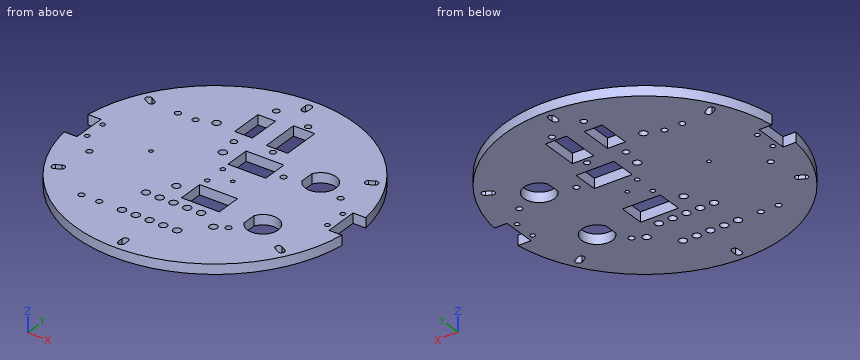
```python
from build123d import *

# Parameters (mm, degrees)
ESQUISSE1_R                     = 71
BOSS_EXTRU_1_DEPTH              = 5
ESQUISSE2_W                     = 33.992340046
ESQUISSE2_H                     = 17
ESQUISSE2_W_2                   = 21.861356716
ENL_V_MAT_EXTRU_1_DEPTH         = 101.533576481
D_GAGEMENT_M21_D                = 2.4
R_P_TITION_LIN_AIRE1_COUNT      = 3
R_P_TITION_LIN_AIRE1_PITCH      = 61
R_P_TITION_LIN_AIRE1_COUNT_DIR2 = 2
R_P_TITION_LIN_AIRE1_PITCH_DIR2 = 11
ESQUISSE7_R                     = 1
ENL_V_MAT_EXTRU_2_DEPTH         = 10
ENL_V_MAT_EXTRU_3_DEPTH         = 101.173599316
D_GAGEMENT_M25_DEPTH            = 5
R_P_TITION_CIRCULAIRE1_COUNT    = 6
ESQUISSE11_R                    = 1.6
ESQUISSE11_R_2                  = 1.5
ESQUISSE11_R_3                  = 1.975
ESQUISSE11_R_4                  = 1
ESQUISSE11_W                    = 19.2
ESQUISSE11_H                    = 12.9
ESQUISSE11_W_2                  = 9
ESQUISSE11_H_2                  = 16.5
ESQUISSE11_W_3                  = 10.8
ESQUISSE11_H_3                  = 19.2
ENL_V_MAT_EXTRU_4_DEPTH         = 101.173599316
ESQUISSE12_R                    = 1.975
ENL_V_MAT_EXTRU_5_DEPTH         = 101.173599316
R_P_TITION_LIN_AIRE3_COUNT      = 5
R_P_TITION_LIN_AIRE3_PITCH      = 7
R_P_TITION_LIN_AIRE3_COUNT_DIR2 = 2
R_P_TITION_LIN_AIRE3_PITCH_DIR2 = 17
ESQUISSE13_R                    = 2
ENL_V_MAT_EXTRU_6_DEPTH         = 101.173599316
R_P_TITION_CIRCULAIRE2_COUNT    = 2
ESQUISSE15_R                    = 1.5
ENL_V_MAT_EXTRU_8_DEPTH         = 10


# Read off the part's stored shape, not the designer's step: Dégagement M25
with BuildPart() as part:
    # Esquisse1 → Boss.-Extru.1 (new body)
    with BuildSketch(Plane.XY):
        Circle(ESQUISSE1_R)
    extrude(amount=BOSS_EXTRU_1_DEPTH)

    # Esquisse2 → Enlèv. mat.-Extru.1 (cut, through all)
    with BuildSketch(Plane.XY.offset(5)):
        with Locations((80.996170023, 0)):
            Rectangle(ESQUISSE2_W, ESQUISSE2_H)
        with Locations((-74.930678358, 0)):
            Rectangle(ESQUISSE2_W_2, ESQUISSE2_H)
    extrude(amount=-ENL_V_MAT_EXTRU_1_DEPTH, mode=Mode.SUBTRACT)

    # Dégagement M21 (through all)
    with Locations(Plane(origin=(0, 0, 0), x_dir=(-1, 0, 0), z_dir=(0, 0, -1))):
        with Locations((-61, -5.5)):
            d_gagement_m21 = Hole(D_GAGEMENT_M21_D / 2)

    # Répétition linéaire1: D_gagement M21 3 × 2
    with Locations(*[(-i * R_P_TITION_LIN_AIRE1_PITCH, j * R_P_TITION_LIN_AIRE1_PITCH_DIR2, 0) for i in range(R_P_TITION_LIN_AIRE1_COUNT) for j in range(R_P_TITION_LIN_AIRE1_COUNT_DIR2) if (i, j) != (0, 0)]):
        add(d_gagement_m21, mode=Mode.SUBTRACT)

    # Esquisse7 → Enlèv. mat.-Extru.2 (cut)
    with BuildSketch(Plane(origin=(0, 0, 0), x_dir=(-1, 0, 0), z_dir=(0, 0, -1))):
        with Locations((32.5, 0)):
            Circle(ESQUISSE7_R)
    extrude(amount=-ENL_V_MAT_EXTRU_2_DEPTH, mode=Mode.SUBTRACT)

    # Esquisse8 → Enlèv. mat.-Extru.3 (cut, through all)
    with BuildSketch(Plane.XY.offset(5)):
        with BuildLine():
            Line((32, 23.940930107), (32, 17.059069893))
            ThreePointArc((32, 17.059069893), (46.8, 20.5), (32, 23.940930107))
        make_face()
        with BuildLine():
            Line((32, -23.940930107), (32, -17.059069893))
            ThreePointArc((32, -17.059069893), (46.8, -20.5), (32, -23.940930107))
        make_face()
    extrude(amount=-ENL_V_MAT_EXTRU_3_DEPTH, mode=Mode.SUBTRACT)

    # Dégagement M25 outline → Dégagement M25 (cut)
    with BuildSketch(Plane.XY):
        with BuildLine():
            Line((54.279215681, -33.185640646), (56.704086811, -34.585640646))
            ThreePointArc((56.704086811, -34.585640646), (58.889727457, -34), (58.304086811, -31.814359354))
            Line((58.304086811, -31.814359354), (55.879215681, -30.414359354))
            ThreePointArc((55.879215681, -30.414359354), (53.693575035, -31), (54.279215681, -33.185640646))
        make_face()
    d_gagement_m25 = extrude(amount=D_GAGEMENT_M25_DEPTH, mode=Mode.SUBTRACT)

    # Répétition circulaire1: Dégagement M25 ×6 about axis
    r_p_tition_circulaire1_axis = Axis((0, 0, 0), (0, 0, 1))
    for i in range(1, R_P_TITION_CIRCULAIRE1_COUNT):
        add(d_gagement_m25.rotate(r_p_tition_circulaire1_axis, i * 360 / R_P_TITION_CIRCULAIRE1_COUNT), mode=Mode.SUBTRACT)

    # Esquisse11 → Enlèv. mat.-Extru.4 (cut, through all)
    with BuildSketch(Plane(origin=(0, 0, 0), x_dir=(-1, 0, 0), z_dir=(0, 0, -1))):
        with Locations((9, 26)):
            Circle(ESQUISSE11_R)
        with Locations((9, 56)):
            Circle(ESQUISSE11_R)
        with Locations((-9, 28.5)):
            Circle(ESQUISSE11_R_2)
        with Locations((-9, 53.5)):
            Circle(ESQUISSE11_R_2)
        with Locations((7.8, 16.45)):
            Circle(ESQUISSE11_R_3)
        with Locations(Location((7.8, -16.45, 0), (0, 0, 180))):
            Circle(ESQUISSE11_R_3)
        with Locations((-9, 0)):
            Circle(ESQUISSE11_R_4)
        with Locations((-9, -16.45)):
            Rectangle(ESQUISSE11_W, ESQUISSE11_H)
        with Locations((-9, 16.45)):
            Rectangle(ESQUISSE11_W, ESQUISSE11_H)
        with Locations((9, 41)):
            Rectangle(ESQUISSE11_W_2, ESQUISSE11_H_2)
        with Locations((-9, 41)):
            Rectangle(ESQUISSE11_W_3, ESQUISSE11_H_3)
    extrude(amount=-ENL_V_MAT_EXTRU_4_DEPTH, mode=Mode.SUBTRACT)

    # Esquisse12 → Enlèv. mat.-Extru.5 (cut, through all)
    with BuildSketch(Plane.XY.offset(5)):
        with Locations((-15, -45)):
            Circle(ESQUISSE12_R)
    enl_v_mat_extru_5 = extrude(amount=-ENL_V_MAT_EXTRU_5_DEPTH, mode=Mode.SUBTRACT)

    # Répétition linéaire3: Enl_v. mat.-Extru.5 5 × 2
    with Locations(*[(i * R_P_TITION_LIN_AIRE3_PITCH, j * R_P_TITION_LIN_AIRE3_PITCH_DIR2, 0) for i in range(R_P_TITION_LIN_AIRE3_COUNT) for j in range(R_P_TITION_LIN_AIRE3_COUNT_DIR2) if (i, j) != (0, 0)]):
        add(enl_v_mat_extru_5, mode=Mode.SUBTRACT)

    # Esquisse13 → Enlèv. mat.-Extru.6 (cut, through all)
    with BuildSketch(Plane(origin=(0, 0, 0), x_dir=(-1, 0, 0), z_dir=(0, 0, -1))):
        with Locations((23.5374475, 33.959943273)):
            Circle(ESQUISSE13_R)
    enl_v_mat_extru_6 = extrude(amount=-ENL_V_MAT_EXTRU_6_DEPTH, mode=Mode.SUBTRACT)

    # Répétition circulaire2: Enlèv. mat.-Extru.6 ×2 about axis
    r_p_tition_circulaire2_axis = Axis((0, 0, 0), (0, 0, 1))
    for i in range(1, R_P_TITION_CIRCULAIRE2_COUNT):
        add(enl_v_mat_extru_6.rotate(r_p_tition_circulaire2_axis, i * 360 / R_P_TITION_CIRCULAIRE2_COUNT), mode=Mode.SUBTRACT)

    # Esquisse15 → Enlèv. mat.-Extru.8 (cut)
    with BuildSketch(Plane.XY.offset(5)):
        with Locations((53.035, 15.040056727)):
            Circle(ESQUISSE15_R)
        with Locations((24.035, 15.040056727)):
            Circle(ESQUISSE15_R)
        with Locations((29.035, -30.959943273)):
            Circle(ESQUISSE15_R)
        with Locations((-35.5374475, -45.040056727)):
            Circle(ESQUISSE15_R)
        with Locations((-26.5374475, -45.040056727)):
            Circle(ESQUISSE15_R)
        with Locations((-41.0374475, 30.959943273)):
            Circle(ESQUISSE15_R)
        with Locations((-32.0374475, 30.959943273)):
            Circle(ESQUISSE15_R)
        with Locations((-53.0374475, -15.040056727)):
            Circle(ESQUISSE15_R)
    extrude(amount=-ENL_V_MAT_EXTRU_8_DEPTH, mode=Mode.SUBTRACT)


solid = part.part
```
For this review, take the finished solid that the model builds, in its own axes (mm). Round coordinates to 2 decimals unless told otherwise and drop trailing zeros. Loops run counter-clockwise (first coordinate to the right, second up) from the corner with the lowest first, then second, coordinate; pieces in that order, holes last.
(1) We need section B-B (y = -51). Give the boundary of the cut face in (x, z), plus the area to 3 significant figures.
Returned:
outline: (-49.4, 0) - (49.4, 0) - (49.4, 5) - (-49.4, 5) - close
area: 494 mm2
(2) Wall thickness on line 1 along X through (y, z) = (39, 2.05); line 2 along Y through (x, z) = (11.5, 4.25); line 3 along X through (y, z) = (17, 3.45): over which ranges is each line inside the solid? List them lowest first.
Returned:
line 1: x = -59.33 to -13.5, -4.5 to 3.6, 14.4 to 59.33
line 2: y = -70.06 to -46.28, -43.72 to -29.28, -26.72 to -22.9, -10 to 10, 22.9 to 31.4, 50.6 to 70.06
line 3: x = -68.93 to -9.7, -5.9 to -0.6, 18.6 to 32.03, 45.97 to 68.93
(3) We need section A-A (z = 2.8). State how many separate pieces and enclosed holes the cut face has, plus the area to 3 significant figures.
Returned:
separate pieces: 1
enclosed holes: 46
area: 14,000 mm2
(4) Clearance check with flat-ended pins moving along their axes: P1, Ø2.5, axis at x = 9, z = 1.5, coming from the -Y side; P2, Ø1.5, axis at x = -2.5, z = 4.5, coming from the +Y side; P3, Ø1.4, axis at x = 0, y = -5.5, coming from the -Z side; P4, Ø2, axis at y = 65.5, z = 3, coming from the -X side. State where each tip first meets the part, or that it passes through.
Returned:
P1: stops at y = -70.58
P2: stops at y = 70.98
P3: passes through
P4: stops at x = -29.68
